The listing builds one solid part. Answer for the finished solid, in the listing's coordinates (mm). A direction names the side the tool comes from. Give positions to 0.01 mm unless a question says otherwise; leave off trailing zeros. Loops run counter-clockwise (first coordinate to the right, second up) from the corner with the lowest first, then second, coordinate; pieces in that order, holes last. Notation, with made-up numbers: (-23.75, 41.25) - (14.25, 41.25) arc R35 ccw to (14.25, 76.25) - close; hole circle Ø8 at (36, -24.5). An arc over 180 degrees is marked (long way). Answer as CSV lines item,"result". Start each with the question number.
1) For a pull along Z with two mould halves and no side action, classify faces 1 (the face through (-47.032, 175, -14)), 2 (the face through (-5, 175, -64.988)), 3 (the face through (-5.706, 41.727, -65.117)) as pulls with the +Z half, pulls with the -Z half, needs draft (parallel to the pull), parting line crosses it, or undercut.
2) Find the intervals of material crossed by line 1 along Z through (x, y) = (11, 178); line 2 along Y through (x, z) = (17, 18.5); line 3 along Y through (x, z) = (-6, 4), in increasing order.
3) A cutting plane is placed at C-C (z = -20.5). Determine the outline of the cut face in (x, y), and give its area (3 significant figures).
4) A cutting plane is placed at D-D (z = 32). Determine the outline of the cut face in (x, y).
5) For faces 4 (the face through (-6, 42, 34.822)), 5 (the face through (-23, 84.639, -23)), 6 (the face through (-30, 0, -8)), determine the directions among +Z, -Z, +X, -X, +Y, -Y from which every point of the face is accessible in a straight line to the end or side of a thin tool.
6) Flat-ended cylindrical pins translate along their axes: pin 1 (15.5 mm diameter, centred on x = 7.5, y = 166.5, fed in from -Z); pin 2 (6 mm diameter, centred on y = 35, z = -43, fed in from -X); pin 3 (9.5 mm diameter, centred on x = -14.5, z = 30, fed in from -Y). Find the tip coordinate at first contact, or state that the pin passes through.
7) A cutting plane is placed at B-B (x = 2). Determine the outline of the cut face in (y, z), and give its area (3 significant figures).
8) A cutting plane is placed at A-A (y = 52.5). Determine the outline of the cut face in (x, z).
```python
from build123d import *

# Parameters (mm, degrees)
LOFT_THIN1_DEPTH         = 84.63920117
BOSS_EXTRUDE1_DEPTH      = 41.359307983
BOSS_EXTRUDE1_DEPTH_BACK = 10.414
SKETCH8_W                = 84.304447576
SKETCH8_H                = 99.8104289
SKETCH16_W               = 83.624271947
SKETCH16_H               = 22.311451813
BOSS_EXTRUDE2_DEPTH      = 76.2


# Read off the part's stored shape, not the designer's step: Loft-Thin1
with BuildPart() as part:
    # Loft-Thin1 outline → Loft-Thin1 (new body)
    with BuildSketch(Plane(origin=(0, 0, 0), x_dir=(1, 0, 0), z_dir=(0, 1, 0))):
        with BuildLine():
            Line((38.170457439, -37.361978489), (9.323951838, 37.81376338))
            ThreePointArc((9.323951838, 37.81376338), (-5.162903092, 67.673974593), (-18.965674378, 37.491451765))
            Line((-18.965674378, 37.491451765), (-50.875746846, -37.361978489))
            Line((-50.875746846, -37.361978489), (38.170457439, -37.361978489))
        make_face()
        with BuildLine():
            ThreePointArc((-15.982812233, 38.011486845), (-5.185335077, 65.133470666), (6.401715759, 38.339296444))
            Line((6.401715759, 38.339296444), (34.475228233, -34.821978489))
            Line((34.475228233, -34.821978489), (-47.031772168, -34.821978489))
            Line((-47.031772168, -34.821978489), (-15.982812233, 38.011486845))
        make_face(mode=Mode.SUBTRACT)
    extrude(amount=LOFT_THIN1_DEPTH)



with BuildPart() as body_2:
    # Sketch8 → Boss-Extrude1 (new, two sides: drawn at the far end of the back side and taken through both)
    with BuildSketch(Plane(origin=(0, 160, 0), x_dir=(1, 0, 0), z_dir=(0, 1, 0)).offset(-BOSS_EXTRUDE1_DEPTH_BACK)):
        with Locations((-4.87954838, 15.083235961)):
            Rectangle(SKETCH8_W, SKETCH8_H)
    extrude(amount=BOSS_EXTRUDE1_DEPTH + BOSS_EXTRUDE1_DEPTH_BACK)


with BuildPart() as part_1:
    add(part.part)

    add(body_2.part)  # Boss-Extrude2 merges body 2
    # Sketch16 → Boss-Extrude2 (add)
    with BuildSketch(Plane(origin=(0, 160, 0), x_dir=(1, 0, 0), z_dir=(0, 1, 0))):
        with Locations((1.894665963, -27.457802507)):
            Rectangle(SKETCH16_W, SKETCH16_H)
    extrude(amount=-BOSS_EXTRUDE2_DEPTH)


solid = part_1.part
```
Ans:
1,face 1,"needs draft"
1,face 2,"pulls with the -Z half"
1,face 3,"undercut"
2,line 1,"-64.99 to 34.82"
2,line 2,"83.8 to 201.36"
2,line 3,"149.59 to 201.36"
3,outline,"(-47.03, 149.59) - (37.27, 149.59) - (37.27, 201.36) - (-47.03, 201.36) - close; (-26.21, 0) - (-23.45, 0) - (-23.45, 84.64) - (-26.21, 84.64) - close; (13.25, 0) - (15.97, 0) - (15.97, 84.64) - (13.25, 84.64) - close"
3,area,"4,830 mm2"
4,outline,"(-48.59, 0) - (-45.83, 0) - (-45.83, 84.64) - (-48.59, 84.64) - close; (-47.03, 149.59) - (-39.92, 149.59) - (-39.92, 83.8) - (33.39, 83.8) - (33.39, 0) - (36.11, 0) - (36.11, 83.8) - (43.71, 83.8) - (43.71, 160) - (37.27, 160) - (37.27, 201.36) - (-47.03, 201.36) - close"
5,face 4,"-Y"
5,face 5,"-Z, -X"
5,face 6,"+Z, -Z, +X, -X, -Y"
6,pin 1,"z = -64.99"
6,pin 2,"x = -22.99"
6,pin 3,"y = 83.8"
7,outline,"(0, -66.31) - (84.64, -66.31) - (84.64, -63.52) - (0, -63.52) - close; (0, 34.82) - (83.8, 34.82) - (83.8, 16.3) - (149.59, 16.3) - (149.59, -64.99) - (201.36, -64.99) - (201.36, 34.82) - (160, 34.82) - (160, 38.61) - (83.8, 38.61) - (83.8, 37.36) - (0, 37.36) - close"
7,area,"7,120 mm2"
8,outline,"(-50.88, 37.36) - (-18.97, -37.49) arc R18.34 ccw (long way) to (9.32, -37.81) - (38.17, 37.36) - close; hole (-47.03, 34.82) - (-15.98, -38.01) arc R15.8 ccw (long way) to (6.4, -38.34) - (34.48, 34.82) - close"
